from build123d import *

# Parameters (mm, degrees)
F0_R        = 31.75
F0_R_2      = 9.525
F1_DEPTH    = 12.7
F2_T1_DEPTH = 12.7
F3_R        = 1.27
F4_R        = 14.1859
F4_R_2      = 9.525
F5_DEPTH    = 5.1308
F6_R        = 14.1859
F6_R_2      = 9.525
F7_DEPTH    = 5.1308


# Not quite as in the source:
# - a fillet or chamfer that OpenCascade refuses, or shapes differently, is made with other operations: its cross-section is extruded or revolved along the edge and cut away or added


with BuildPart() as f1:
    # F0 (on Front) → F1 (new body)
    with BuildSketch(Plane.XZ):
        with BuildLine():
            Line((19.05, 12.2440905122), (19.05, 31.75))
            ThreePointArc((19.05, 31.75), (0, 50.8), (-19.05, 31.75))
            Line((-19.05, 31.75), (-19.05, 12.2440905122))
            ThreePointArc((-19.05, 12.2440905122), (-19.900738686, 9.0690905122), (-22.225, 6.7448291982))
            ThreePointArc((-22.225, 6.7448291982), (-29.6221228011, 1.3910974586), (-35.7691769709, -5.3612054307))
            ThreePointArc((-35.7691769709, -5.3612054307), (-41.1209561154, -14.8719234463), (-43.9940905122, -25.4))
            Line((-43.9940905122, -25.4), (-50.8, -25.4))
            Line((-50.8, -25.4), (-50.8, -38.1))
            Line((-50.8, -38.1), (-43.9940905122, -38.1))
            ThreePointArc((-43.9940905122, -38.1), (0, -76.2), (43.9940905122, -38.1))
            Line((43.9940905122, -38.1), (50.8, -38.1))
            Line((50.8, -38.1), (50.8, -25.4))
            Line((50.8, -25.4), (43.9940905122, -25.4))
            ThreePointArc((43.9940905122, -25.4), (41.1209561154, -14.8719234463), (35.7691769709, -5.3612054307))
            ThreePointArc((35.7691769709, -5.3612054307), (29.6221228011, 1.3910974586), (22.225, 6.7448291982))
            ThreePointArc((22.225, 6.7448291982), (19.900738686, 9.0690905122), (19.05, 12.2440905122))
        make_face()
        with Locations((0, -31.75)):
            Circle(F0_R, mode=Mode.SUBTRACT)
        with Locations((0, 31.75)):
            Circle(F0_R_2, mode=Mode.SUBTRACT)
    extrude(amount=F1_DEPTH)

    # F2: fillet of radius 8.89 on 4 edges, made by hand

    # F2_s2 → F2_t1 (join)
    with BuildSketch(Plane.XZ):
        with BuildLine():
            ThreePointArc((-50.8, -25.4), (-45.6782912458, -23.5470098171), (-42.5985100968, -19.0547474412))
            ThreePointArc((-42.5985100968, -19.0547474412), (-43.4123850712, -22.2018419352), (-43.9940905122, -25.4))
            Line((-43.9940905122, -25.4), (-50.8, -25.4))
        make_face()
        with BuildLine():
            ThreePointArc((50.8, -25.4), (45.6782912458, -23.5470098171), (42.5985100968, -19.0547474412))
            ThreePointArc((42.5985100968, -19.0547474412), (43.4123850712, -22.2018419352), (43.9940905122, -25.4))
            Line((43.9940905122, -25.4), (50.8, -25.4))
        make_face()
        with BuildLine():
            ThreePointArc((-42.5985100968, -44.4452525588), (-45.6782912458, -39.9529901829), (-50.8, -38.1))
            Line((-50.8, -38.1), (-43.9940905122, -38.1))
            ThreePointArc((-43.9940905122, -38.1), (-43.4123850712, -41.2981580648), (-42.5985100968, -44.4452525588))
        make_face()
        with BuildLine():
            ThreePointArc((50.8, -38.1), (45.6782912458, -39.9529901829), (42.5985100968, -44.4452525588))
            ThreePointArc((42.5985100968, -44.4452525588), (43.4123850712, -41.2981580648), (43.9940905122, -38.1))
            Line((43.9940905122, -38.1), (50.8, -38.1))
        make_face()
    extrude(amount=F2_T1_DEPTH)

    # F3
    f3_edges = [f1.edges().sort_by_distance(p)[0] for p in [
        (-50.8, -6.35, -25.4),
        (-50.8, -6.35, -38.1),
        (50.8, -6.35, -25.4),
        (50.8, -6.35, -38.1),
    ]]
    fillet(f3_edges, radius=F3_R)

    # F4 (on face) → F5 (cut)
    with BuildSketch(Plane.XZ.offset(12.7)):
        with Locations((0, 31.75)):
            Circle(F4_R)
        with Locations((0, 31.75)):
            Circle(F4_R_2, mode=Mode.SUBTRACT)
    extrude(amount=-F5_DEPTH, mode=Mode.SUBTRACT)

    # F6 (on face) → F7 (cut)
    with BuildSketch(Plane(origin=(0, 0, 0), x_dir=(-1, 0, 0), z_dir=(0, 1, 0))):
        with Locations((0, 31.75)):
            Circle(F6_R)
        with Locations((0, 31.75)):
            Circle(F6_R_2, mode=Mode.SUBTRACT)
    extrude(amount=-F7_DEPTH, mode=Mode.SUBTRACT)


solid = f1.part
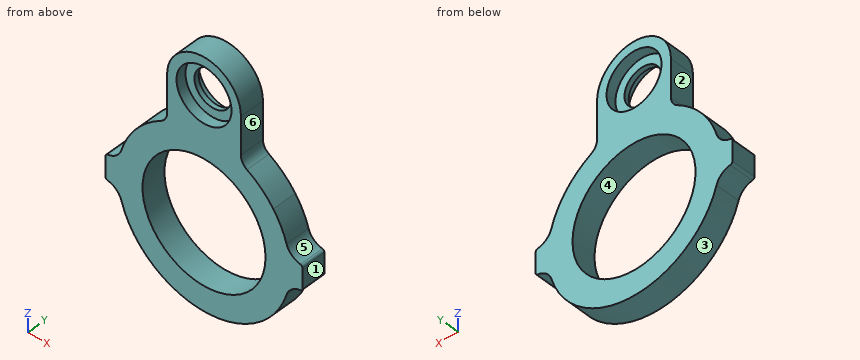
Can you work these out from the model? Positions are in its coordinate system, mm. Face numbers are marked on the shaded views. A direction names the side the tool comes from. Coordinates: 2 decimals unless noted, no trailing zeros. Write each loop counter-clockwise with the first axis right and the second up, starting at its lowest first coordinate (ties: lowest second). Pieces come first, ordered by that corner, then holes. Notation, with made-up numbers: (45, 73.5) -> (78, 73.5) arc R28 cw to (78, 107.5) -> close; hole circle Ø2 at (-15, 67.5). An arc over 180 degrees is marked (long way). Write each question's results on one line, items separated by ' | '. Start each with the question number.
Q1. Imagine slicing it at B-B (x = 0). Write out the boundary of the cut face in (y, z) (3 decimals).
Q2. On a 3-axis mill with a long thin cutter (end or side, diameter ignored), from which of +Z, -Z, +X, -X, +Y, -Y can I reach the whole of each face in a straight line? I mean the marked faces 1 and 2. Say none if no direction works.
Q3. Imagine slicing it at D-D (x = -26.5). Write out the boundary of the cut face in (y, z), then the cut area to 3 significant figures.
Q4. We'd pull the mould along Z, two halves only. Please class the marked faces 3, 4, 5 and 6: +Z half, -Z half, draft (parallel to the pull), parting line (faces both ways), or undercut.
Q5. If I drill on probe 1 along X at (y, z) = (-7.25, 31.5); probe 2 along Z at (x, y) = (-6.5, -11); probe 3 along Z at (x, y) = (-3, -10.75), over which ranges is the centre line in solid material (lowest first)?
Q6. I'm going to push flat-ended pins straight in: pin 1 (3 mm diameter, centred on x = -19, y = -9, fed in from -Z); pin 2 (1.5 mm diameter, centred on y = -7, z = 25.5, fed in from +X); pin 3 (1.5 mm diameter, centred on y = -5.5, z = -6, fed in from +X); pin 4 (15 mm diameter, centred on x = 0, z = 31.75, fed in from -Y). Where does each tip first touch, or does it pass through?
Q7. Imagine slicing it at A-A (z = -31.75). Write out the boundary of the cut face in (x, y).
Q8. Imagine slicing it at C-C (y = -3.5). Write out the boundary of the cut face in (x, z) (3 decimals), then the cut area to 3 significant figures.
Taken from the geometry:
1) outline: (-12.7, -76.2) -> (0, -76.2) -> (0, -63.5) -> (-12.7, -63.5) -> close; (-12.7, 0) -> (0, 0) -> (0, 17.564) -> (-5.131, 17.564) -> (-5.131, 22.225) -> (-7.569, 22.225) -> (-7.569, 17.564) -> (-12.7, 17.564) -> close; (-12.7, 45.936) -> (-7.569, 45.936) -> (-7.569, 41.275) -> (-5.131, 41.275) -> (-5.131, 45.936) -> (0, 45.936) -> (0, 50.8) -> (-12.7, 50.8) -> close
2) face 1: +Z, -Z, +X, +Y, -Y | face 2: +Z, -X, +Y, -Y
3) outline: (-12.7, -67.44) -> (0, -67.44) -> (0, -49.24) -> (-12.7, -49.24) -> close; (-12.7, -14.26) -> (0, -14.26) -> (0, 3.94) -> (-12.7, 3.94) -> close | area: 462 mm^2
4) face 3: -Z half | face 4: undercut | face 5: +Z half | face 6: draft
5) probe 1: x = -19.05 to -9.52, 9.52 to 19.05 | probe 2: z = -75.72 to -62.83, -0.67 to 19.14, 44.36 to 49.66 | probe 3: z = -76.1 to -63.36, -0.14 to 17.88, 45.62 to 50.56
6) pin 1: stops at z = -72.61 | pin 2: stops at x = 19.05 | pin 3: stops at x = 36.75 | pin 4: passes through
7) outline: (-50.8, -12.7) -> (-31.75, -12.7) -> (-31.75, 0) -> (-50.8, 0) -> close; (31.75, -12.7) -> (50.8, -12.7) -> (50.8, 0) -> (31.75, 0) -> close
8) outline: (-50.8, -36.949) arc R1.27 ccw to (-49.729, -38.204) arc R8.89 cw to (-42.599, -44.445) arc R44.45 ccw to (42.599, -44.445) arc R8.89 cw to (49.729, -38.204) arc R1.27 ccw to (50.8, -36.949) -> (50.8, -26.551) arc R1.27 ccw to (49.729, -25.296) arc R8.89 cw to (42.599, -19.055) arc R44.45 ccw to (22.225, 6.745) arc R6.35 cw to (19.05, 12.244) -> (19.05, 31.75) arc R19.05 ccw to (-19.05, 31.75) -> (-19.05, 12.244) arc R6.35 cw to (-22.225, 6.745) arc R44.45 ccw to (-42.599, -19.055) arc R8.89 cw to (-49.729, -25.296) arc R1.27 ccw to (-50.8, -26.551) -> close; hole circle Ø63.5 at (0, -31.75); hole circle Ø28.372 at (0, 31.75) | area: 3,960 mm^2
